The drawing under review shows one solid part. Ordinate dimensions are in mm from its lowest x, y, z. Give positions to 0.01 mm unless a question says otherwise; leave off trailing zeros. Loops run counter-clockwise (first coordinate to the right, second up) from the corner with the lowest first, then second, coordinate; pieces in that order, holes last. Notation, with made-up numbers: M 62.25,-27 L 72.25,-27 A20 cw 72.25,-14 Z; hole C 26.25,79.25 d1. An arc over 180 degrees is marked long. Put each result on its own line as item: value. Start each with the question number.
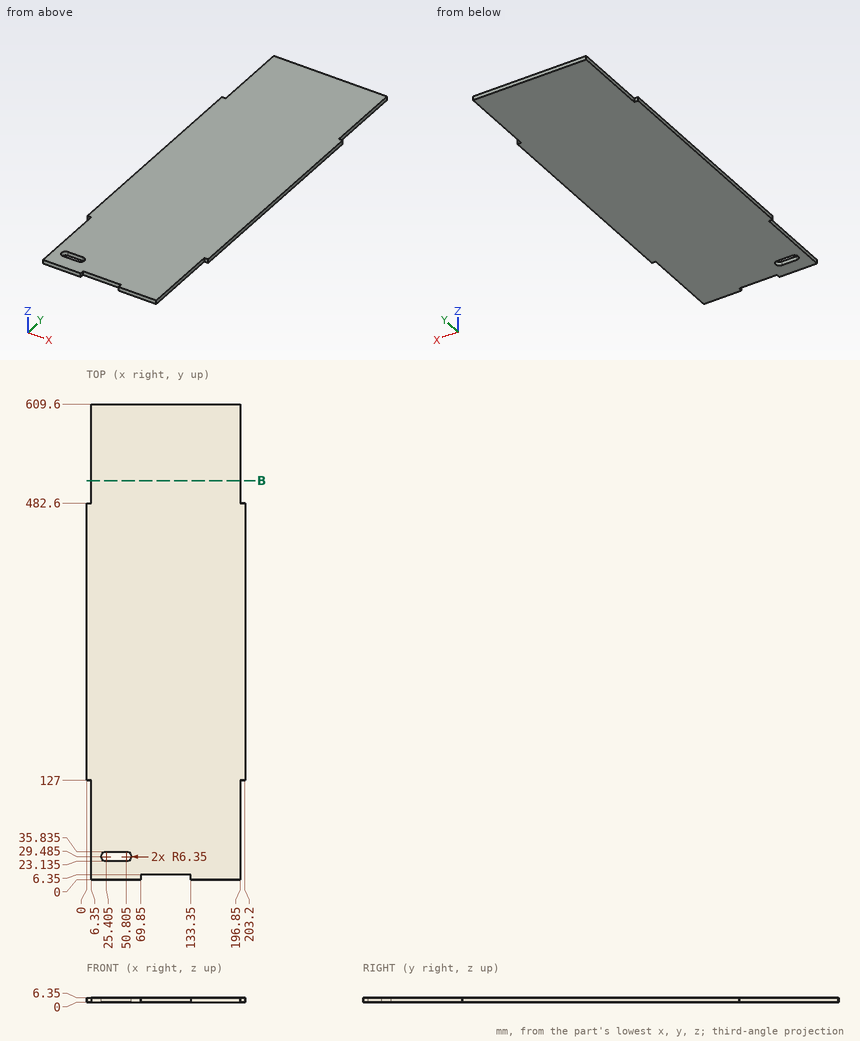
Item 1: To check wall thickness, follow L1, parallel to Y at x = 25.5, z = 1 (1 decimal); L2, parallel to Y at x = 72, z = 5.25; L3, parallel to Y at x = 23.5, z = 3.25. State the ranges of each line that lie inside material, in increasing order. Write a range as [from, to].
Item 2: Consider section B-B, the plane y = 511.5. Write out the cut boundary in (x, z), plus the area to 3 significant figures.
Item 3: Clearance check with flat-ended pins moving along their axes: pin 1 Ø3 at (x, y) = (100.5, 497.5) entering from -Z; pin 2 Ø3 at (x, z) = (201.5, 3) entering from -Y; pin 3 Ø3 at (x, z) = (3.5, 2) entering from +Y; pin 4 Ø3 at (y, z) = (560.5, 3) entering from -X. State where each tip first meets the part, or that it passes through.
Report:
1. L1: [0, 23.1], [35.8, 609.6]
1. L2: [6.35, 609.6]
1. L3: [0, 23.43], [35.54, 609.6]
2. outline: M 6.35,0 L 196.85,0 L 196.85,6.35 L 6.35,6.35 Z
2. area: 1,210 mm²
3. pin 1: z = 0
3. pin 2: y = 127
3. pin 3: y = 482.6
3. pin 4: x = 6.35
